```python
from build123d import *

# Parameters (mm, degrees)
BOSS_EXTRUDE1_DEPTH = 8.89
FILLET1_R           = 4.318


with BuildPart() as part:
    # Sketch1 → Boss-Extrude1 (new body)
    with BuildSketch(Plane.XY):
        Polygon((-19.4945, 0.635), (-30.1625, 0.635), (-30.1625, -12.065), (-21.2725, -12.065), (30.1625, 12.065), (-14.2875, 12.065), (-14.2875, 4.445), align=None)
    extrude(amount=BOSS_EXTRUDE1_DEPTH)

    # Fillet1
    fillet1_edges = [part.edges().sort_by_distance(p)[0] for p in [
        (-30.1625, -5.715, 8.89),
        (-30.1625, -5.715, 0),
    ]]
    fillet(fillet1_edges, radius=FILLET1_R)


solid = part.part
```
Here's how the part is built. I have some questions about the finished solid (model axes, mm). A direction names the side the tool comes from. Give positions to 0.01 mm unless a question says otherwise; leave off trailing zeros. Loops run counter-clockwise (first coordinate to the right, second up) from the corner with the lowest first, then second, coordinate; pieces in that order, holes last. Notation, with made-up numbers: M 59,82.25 L 107,82.25 A17 cw 107,99.25 Z; hole C 35,26.5 d11. An arc over 180 degrees is marked long. Return JSON: item names as keys, results as strings.
Item 1: Please list where these lines run through material, in increasing order: line 1 (Y direction, x = -22, z = 6) (3 decimals); line 2 (X direction, y = -10.25, z = 7.5); line 3 (Z direction, x = -26, y = -3).
A:
{"line 1": "y = -12.065 to 0.635", "line 2": "x = -29.02 to -17.4", "line 3": "z = 0 to 8.89"}
Item 2: Imagine slicing it at C-C on y = -9. List the corners of the cut face in (x, z) for me, then the cut area to 3 significant figures.
A:
{"outline": "M -30.16,4.32 A4.32 ccw -25.84,0 L -14.74,0 L -14.74,8.89 L -25.84,8.89 A4.32 ccw -30.16,4.57 Z", "area": "129 mm^2"}
Item 3: Imagine slicing it at D-D on z = 8. List the corners of the cut face in (x, y) for me (1 decimal).
A:
{"outline": "M -28.5,-12.1 L -21.3,-12.1 L 30.2,12.1 L -14.3,12.1 L -14.3,4.4 L -19.5,0.6 L -28.5,0.6 Z"}
Item 4: Imagine slicing it at A-A on z = 3.5. List the corners of the cut face in (x, y) for me (1 decimal).
A:
{"outline": "M -30.1,-12.1 L -21.3,-12.1 L 30.2,12.1 L -14.3,12.1 L -14.3,4.4 L -19.5,0.6 L -30.1,0.6 Z"}
Item 5: I'm going to push flat-ended pins straight in: pin 1 Ø8 at (x, y) = (6, -2) entering from -Z; pin 2 Ø4 at (x, z) = (13.5, 4) entering from -Y; pin 3 Ø5 at (y, z) = (7, 5.5) entering from -X. Where does each tip first touch, or does it pass through?
A:
{"pin 1": "stops at z = 0", "pin 2": "stops at y = 3.31", "pin 3": "stops at x = -14.29"}
Item 6: Imagine slicing it at B-B on x = -24.5. List the corners of the cut face in (y, z) for me (3 decimals), then the cut area to 3 significant figures.
A:
{"outline": "M -12.065,0 L 0.635,0 L 0.635,8.89 L -12.065,8.89 Z", "area": "113 mm^2"}
Item 7: On a 3-axis mill with a long thin cutter (end or side, diameter ignored), from which of +Z, -Z, +X, -X, +Y, -Y can I reach the whole of each face in a straight line? I mean faces 1 (the flat face through (-14.288, 8, 4)), 2 (the flat face through (8, 12.065, 4)). Say none if no direction works.
A:
{"face 1": "+Z, -Z, -X, +Y", "face 2": "+Z, -Z, +X, -X, +Y"}
